Check sheet for the modelled part. Datum: model origin and axes. Units: mm. A direction names the side the tool comes from. Give positions to 0.01 mm unless a question says otherwise; leave off trailing zeros. Order: outer loops, then holes, each group sorted by start corner. A loop starts at its lowest first (then second) coordinate and runs counter-clockwise, first axis right, second up.
Item 1: Access from +Z, -Z, +X, -X, +Y, -Y to the whole of each face (thin tool, end or side, straight path). Record for faces 4 (the flat face through (-22.205, 60, 3)), 5 (the flat face through (-18, 54.731, 3)), 6 (the flat face through (-19.825, -1, -4)), 7 (the flat face through (23.138, -1, -4)).
Item 2: Sectioned sample at A-A on z = -2.25. Record the boundary of the cut face in (x, y), and give its area (3 significant figures).
Item 3: Release check for a two-part mould opening along X. For faces 1 (the flat face through (-18, 60, 5)), 2 (the flat face through (-13.879, 60, 3)), 3 (the cylindrical face through (-26.958, 63.786, 0.986)) record: released by +X, released by -X, zero draft, split by the parting line, or undercut.
Item 4: Gauge pin test, flat ends, axial feed: P1, Ø4.5, axis at y = -15, z = -6.5, coming from the +X side; P2, Ø1.3, axis at x = 21.5, z = -2.5, coming from the +Y side; P3, Ø2, axis at x = 10, y = -35, coming from the +Z side; P4, Ø1.5, axis at x = -18, z = 2.5, coming from the -Y side. Record the tip position at first contact, or that the pin passes through.
Item 5: Sectioned sample at C-C on y = 62.2. Record the boundary of the cut face in (x, z), and give its area (3 significant figures).
Item 6: Sectioned sample at B-B on x = 26.75. Record the boundary of the cut face in (y, z), and give its area (3 significant figures).
Item 7: Material ranges on line 1 along Y through (x, z) = (26.75, 1.1); line 2 along X through (y, z) = (-15.5, -5.25); line 3 along Z through (x, y) = (-18, -53), recorded low to high.
Item 8: Sectioned sample at D-D on y = -31.5. Record the boundary of the cut face in (x, z), and give its area (3 significant figures).
from build123d import *

# Parameters (mm, degrees)
SKETCH1_W           = 58.6
SKETCH1_H           = 129.8
SKETCH1_R           = 1.6
BOSS_EXTRUDE1_DEPTH = 2
SKETCH2_W           = 4.296297389
SKETCH2_H           = 105.080273626
SKETCH2_W_2         = 3.938272606
BOSS_EXTRUDE2_DEPTH = 9
SKETCH3_W           = 8.325714973
SKETCH3_H           = 11.044315781
BOSS_EXTRUDE3_DEPTH = 3


with BuildPart() as part:
    # Sketch1 → Boss-Extrude1 (new body)
    with BuildSketch(Plane.XY):
        Rectangle(SKETCH1_W, SKETCH1_H)
        with Locations((-26.75, 62.2)):
            Circle(SKETCH1_R, mode=Mode.SUBTRACT)
        with Locations((26.75, 62.2)):
            Circle(SKETCH1_R, mode=Mode.SUBTRACT)
        with Locations((-26.75, -62.2)):
            Circle(SKETCH1_R, mode=Mode.SUBTRACT)
        with Locations((26.75, -62.2)):
            Circle(SKETCH1_R, mode=Mode.SUBTRACT)
    extrude(amount=BOSS_EXTRUDE1_DEPTH)

    # Sketch2 → Boss-Extrude2 (add)
    with BuildSketch(Plane(origin=(0, 0, 0), x_dir=(-1, 0, 0), z_dir=(0, 0, -1))):
        with Locations((-20.989773544, 0)):
            Rectangle(SKETCH2_W, SKETCH2_H)
        with Locations((21.79418795, 0)):
            Rectangle(SKETCH2_W_2, SKETCH2_H)
    extrude(amount=BOSS_EXTRUDE2_DEPTH)

    # Sketch3 → Boss-Extrude3 (add)
    with BuildSketch(Plane.XY.offset(2)):
        with Locations((-18.042212682, 60.253196822)):
            Rectangle(SKETCH3_W, SKETCH3_H)
    extrude(amount=BOSS_EXTRUDE3_DEPTH)


solid = part.part
Report:
1. face 4: +Z, -X, +Y, -Y
1. face 5: +Z, +X, -X, -Y
1. face 6: -Z, +Y, -Y
1. face 7: -Z, +X, +Y, -Y
2. outline: (-23.76, -52.54) - (-19.83, -52.54) - (-19.83, 52.54) - (-23.76, 52.54) - close; (18.84, -52.54) - (23.14, -52.54) - (23.14, 52.54) - (18.84, 52.54) - close
2. area: 865 mm2
3. face 1: zero draft
3. face 2: released by +X
3. face 3: undercut
4. P1: stops at x = 23.14
4. P2: stops at y = 52.54
4. P3: stops at z = 2
4. P4: stops at y = -64.9
5. outline: (-29.3, 0) - (-28.35, 0) - (-28.35, 2) - (-29.3, 2) - close; (-25.15, 0) - (25.15, 0) - (25.15, 2) - (-13.88, 2) - (-13.88, 5) - (-22.21, 5) - (-22.21, 2) - (-25.15, 2) - close; (28.35, 0) - (29.3, 0) - (29.3, 2) - (28.35, 2) - close
5. area: 129 mm2
6. outline: (-64.9, 0) - (-63.8, 0) - (-63.8, 2) - (-64.9, 2) - close; (-60.6, 0) - (60.6, 0) - (60.6, 2) - (-60.6, 2) - close; (63.8, 0) - (64.9, 0) - (64.9, 2) - (63.8, 2) - close
6. area: 247 mm2
7. line 1: y = -64.9 to -63.8, -60.6 to 60.6, 63.8 to 64.9
7. line 2: x = -23.76 to -19.83, 18.84 to 23.14
7. line 3: z = 0 to 2
8. outline: (-29.3, 0) - (-23.76, 0) - (-23.76, -9) - (-19.83, -9) - (-19.83, 0) - (18.84, 0) - (18.84, -9) - (23.14, -9) - (23.14, 0) - (29.3, 0) - (29.3, 2) - (-29.3, 2) - close
8. area: 191 mm2
